```python
from build123d import *

# Parameters (mm, degrees)
RESSALTO_EXTRUS_O1_DEPTH   = 60
ESBO_O2_R                  = 9
CORTE_EXTRUS_O1_DEPTH      = 13
CORTE_EXTRUS_O1_DEPTH_BACK = 9
ESBO_O3_R                  = 1.65
CORTE_EXTRUS_O2_DEPTH      = 37.3
ESBO_O4_R                  = 11.05
CORTE_EXTRUS_O3_DEPTH      = 7
CORTE_EXTRUS_O5_START      = 6
ESBO_O7_R                  = 5.25
CORTE_EXTRUS_O5_DEPTH      = 10
ESBO_O7_2_R                = 5.25
CORTE_EXTRUS_O7_DEPTH      = 1
FILETE1_R                  = 6


with BuildPart() as part:
    # Esboço1 → Ressalto-extrusão1 (new body)
    with BuildSketch(Plane.XY):
        Polygon((0, 0), (6, 0), (10.367642811, 12), (49, 12), (49, 20), (0, 20), align=None)
    extrude(amount=RESSALTO_EXTRUS_O1_DEPTH)

    # Esboço2 → Corte-extrusão1 (cut, two sides)
    with BuildSketch(Plane.XZ.offset(-12)) as corte_extrus_o1_sk:
        with Locations((21.3, 30)):
            Circle(ESBO_O2_R)
        with BuildLine():
            Line((21.3, 15), (10.367642811, 15))
            Line((10.367642811, 15), (6, 4))
            Line((6, 4), (0, 4))
            Line((0, 4), (0, 0))
            Line((0, 0), (49, 0))
            Line((49, 0), (49, 60))
            Line((49, 60), (0, 60))
            Line((0, 60), (0, 56))
            Line((0, 56), (6, 56))
            Line((6, 56), (10.367642811, 45))
            Line((10.367642811, 45), (21.3, 45))
            ThreePointArc((21.3, 45), (36.3, 30), (21.3, 15))
        make_face()
    extrude(amount=CORTE_EXTRUS_O1_DEPTH, mode=Mode.SUBTRACT)
    extrude(corte_extrus_o1_sk.sketch, amount=-CORTE_EXTRUS_O1_DEPTH_BACK, mode=Mode.SUBTRACT)

    # Esboço3 → Corte-extrusão2 (cut, through all)
    with BuildSketch(Plane.ZY):
        with Locations((50, 10)):
            Circle(ESBO_O3_R)
        with Locations((10, 10)):
            Circle(ESBO_O3_R)
    extrude(amount=-CORTE_EXTRUS_O2_DEPTH, mode=Mode.SUBTRACT)

    # Esboço4 → Corte-extrusão3 (cut)
    with BuildSketch(Plane(origin=(0, 20, 0), x_dir=(1, 0, 0), z_dir=(0, 1, 0))):
        with Locations((21.3, -30)):
            Circle(ESBO_O4_R)
    extrude(amount=-CORTE_EXTRUS_O3_DEPTH, mode=Mode.SUBTRACT)

    # Esboço7 → Corte-extrusão5 (cut)
    with BuildSketch(Plane(origin=(0, 0, 0), x_dir=(0, 0, -1), z_dir=(1, 0, 0)).offset(CORTE_EXTRUS_O5_START)):
        with Locations((-50, 10)):
            Circle(ESBO_O7_R)
        with Locations((-10, 10)):
            Circle(ESBO_O7_R)
    extrude(amount=CORTE_EXTRUS_O5_DEPTH, mode=Mode.SUBTRACT)

    # Esboço7<2> → Corte-extrusão7 (cut)
    with BuildSketch(Plane(origin=(0, 0, 0), x_dir=(0, 0, -1), z_dir=(1, 0, 0))):
        with Locations((-50, 10)):
            Circle(ESBO_O7_2_R)
        with Locations((-10, 10)):
            Circle(ESBO_O7_2_R)
    extrude(amount=CORTE_EXTRUS_O7_DEPTH, mode=Mode.SUBTRACT)

    # Filete1
    filete1_edges = [part.edges().sort_by_distance(p)[0] for p in [
        (3, 0, 4),
        (3, 0, 56),
        (3, 20, 4),
        (3, 20, 56),
    ]]
    fillet(filete1_edges, radius=FILETE1_R)


solid = part.part
```
Geometry check sheet. Reference: the model listing, model coordinates, mm. A direction names the side the tool comes from. Coordinates: 2 decimals unless noted, no trailing zeros. Loops run counter-clockwise (first coordinate to the right, second up) from the corner with the lowest first, then second, coordinate; pieces in that order, holes last. Notation, with made-up numbers: (-40, 3.25) -> (-26, 3.25) arc R29 cw to (-26, 28.25) -> close; hole circle Ø8 at (71.5, -36.5). An arc over 180 degrees is marked (long way). Put each result on its own line as item: value.
1) Cross-section at A-A on z = 30. Record the boundary of the cut face in (x, y).
Result set:
outline: (0, 0) -> (6, 0) -> (10.37, 12) -> (12.3, 12) -> (12.3, 13) -> (10.25, 13) -> (10.25, 20) -> (0, 20) -> close; (30.3, 12) -> (36.3, 12) -> (36.3, 20) -> (32.35, 20) -> (32.35, 13) -> (30.3, 13) -> close
2) Thickness scan on line 1 (Z direction, x = 3, y = 9); line 2 (Y direction, x = 3.5, z = 50); line 3 (X direction, y = 18, z = 30). Record the ranges inside material, lowest first.
Result set:
line 1: z = 4 to 8.69, 11.31 to 48.69, 51.31 to 56
line 2: y = 0 to 8.35, 11.65 to 20
line 3: x = 0 to 10.25, 32.35 to 36.3
3) Gauge pin test, flat ends, axial feed: pin 1 Ø8.5 at (y, z) = (10, 50) entering from -X; pin 2 Ø2.5 at (x, y) = (13.5, 18) entering from +Z; pin 3 Ø9 at (x, y) = (18, 16) entering from -Z. Record the tip position at first contact, or that the pin passes through.
Result set:
pin 1: stops at x = 1
pin 2: stops at z = 45
pin 3: stops at z = 15
4) Tool access check on faces 5 (the flat face through (1, 10, 48)), 6 (the cylindrical face through (31.51, 16.55, 34.23)), 7 (the flat face through (16, 16, 45)). Record the directions out of +Z, -Z, +X, -X, +Y, -Y that give a thin tool (end or side, any length) a straight path to the whole face; none if there is none.
Result set:
face 5: -X
face 6: +Y
face 7: +Z, +X, +Y, -Y
5) Cross-section at B-B on x = 27. Record the boundary of the cut face in (y, z).
Result set:
outline: (12, 16.13) -> (20, 16.13) -> (20, 20.53) -> (13, 20.53) -> (13, 23.04) -> (12, 23.04) -> close; (12, 36.96) -> (13, 36.96) -> (13, 39.47) -> (20, 39.47) -> (20, 43.87) -> (12, 43.87) -> close
6) Release check for a two-part mould opening along Y. For faces 1 (the cylindrical face through (29.884, 12.493, 32.703)), 2 (the cylindrical face through (7.2, 11.6, 45)), 3 (the cylindrical face through (3.287, 1.711, 5.804)), 4 (the cylindrical face through (7.172, 10.231, 15.245)) record: released by +Y, released by -Y, zero draft, split by the parting line, or undercut.
Result set:
face 1: zero draft
face 2: undercut
face 3: released by -Y
face 4: undercut
7) Cross-section at C-C on y = 10. Record the boundary of the cut face in (x, z), plus the area to 3 significant figures.
Result set:
outline: (0, 4) -> (6, 4) -> (6.3, 4.75) -> (6, 4.75) -> (6, 8.35) -> (1, 8.35) -> (1, 4.75) -> (0, 4.75) -> close; (0, 15.25) -> (1, 15.25) -> (1, 11.65) -> (6, 11.65) -> (6, 15.25) -> (9.64, 15.25) -> (9.64, 44.75) -> (6, 44.75) -> (6, 48.35) -> (1, 48.35) -> (1, 44.75) -> (0, 44.75) -> close; (0, 55.25) -> (1, 55.25) -> (1, 51.65) -> (6, 51.65) -> (6, 55.25) -> (6.3, 55.25) -> (6, 56) -> (0, 56) -> close
area: 366 mm^2
8) Cross-section at D-D on z = 46. Record the boundary of the cut face in (x, y).
Result set:
outline: (0, 0) -> (6, 0) -> (8.4, 6.6) -> (6, 6.6) -> (6, 13.4) -> (9.97, 13.4) -> (9.97, 20) -> (0, 20) -> (0, 13.4) -> (1, 13.4) -> (1, 6.6) -> (0, 6.6) -> close
